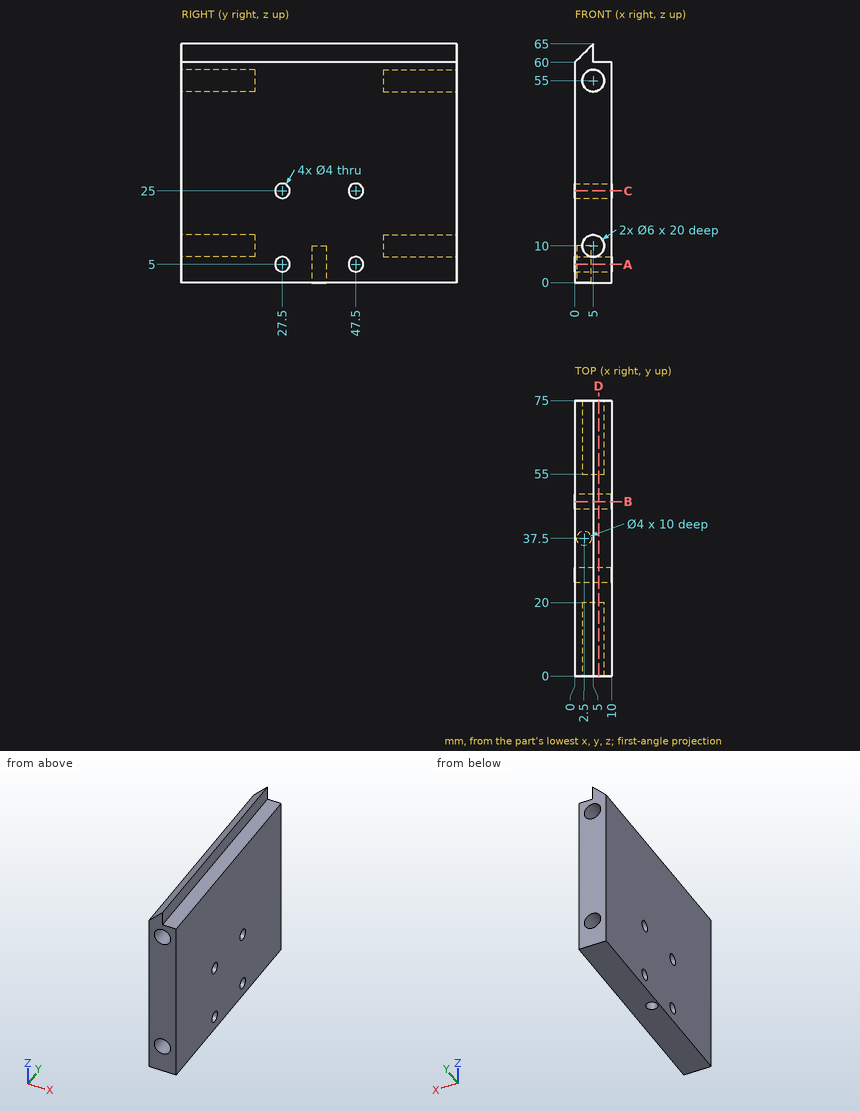
Can you work these out from the drawing? Everything is in mm from the part's minimum corner. Give positions to 0.01 mm unless a question says otherwise; leave off trailing zeros. Loops run counter-clockwise (first coordinate to the right, second up) from the corner with the lowest first, then second, coordinate; pieces in that order, holes last. Notation, with made-up numbers: (-18, 26) -> (33, 26) arc R12 ccw to (33, 30) -> close; hole circle Ø7 at (52.5, 48). An arc over 180 degrees is marked (long way). Put each result on its own line as item: value.
(1) Please list where these lines run through material, in increasing order: probe 1 along Z at (x, y) = (7, 47.5); probe 2 along Z at (x, y) = (4.25, 26); probe 3 along Y at (x, z) = (2, 6). Write a range as [from, to].
Computed:
probe 1: [0, 3], [7, 23], [27, 60]
probe 2: [0, 3.68], [6.32, 23.68], [26.32, 64.25]
probe 3: [0, 25.77], [29.23, 35.56], [39.44, 45.77], [49.23, 75]
(2) Imagine slicing it at C-C on z = 25. Write out the boundary of the cut face in (x, y), plus the area to 3 significant figures.
Computed:
outline: (0, 0) -> (10, 0) -> (10, 25.5) -> (0, 25.5) -> close; (0, 29.5) -> (10, 29.5) -> (10, 45.5) -> (0, 45.5) -> close; (0, 49.5) -> (10, 49.5) -> (10, 75) -> (0, 75) -> close
area: 670 mm^2
(3) Imagine slicing it at A-A on z = 5. Write out the boundary of the cut face in (x, y).
Computed:
outline: (0, 0) -> (10, 0) -> (10, 25.5) -> (0, 25.5) -> close; (0, 29.5) -> (10, 29.5) -> (10, 45.5) -> (0, 45.5) -> close; (0, 49.5) -> (10, 49.5) -> (10, 75) -> (0, 75) -> close; hole circle Ø4 at (2.5, 37.5)
(4) I'm going to push flat-ended pins straight in: pin 1 Ø1.5 at (x, y) = (8, 55.5) entering from +Z; pin 2 Ø1.8 at (x, z) = (4, 11) entering from -Y; pin 3 Ø3 at (x, z) = (4.5, 54.5) entering from +Y. Where does each tip first touch, or does it pass through?
Computed:
pin 1: z = 60
pin 2: y = 20
pin 3: y = 55
(5) Imagine slicing it at B-B on y = 47.5. Write out the boundary of the cut face in (x, z).
Computed:
outline: (0, 0) -> (10, 0) -> (10, 3) -> (0, 3) -> close; (0, 7) -> (10, 7) -> (10, 23) -> (0, 23) -> close; (0, 27) -> (10, 27) -> (10, 60) -> (5, 60) -> (5, 65) -> (0, 60) -> close
(6) Imagine slicing it at D-D on x = 6.5. Write out the boundary of the cut face in (y, z).
Computed:
outline: (0, 0) -> (75, 0) -> (75, 7.4) -> (55, 7.4) -> (55, 12.6) -> (75, 12.6) -> (75, 52.4) -> (55, 52.4) -> (55, 57.6) -> (75, 57.6) -> (75, 60) -> (0, 60) -> (0, 57.6) -> (20, 57.6) -> (20, 52.4) -> (0, 52.4) -> (0, 12.6) -> (20, 12.6) -> (20, 7.4) -> (0, 7.4) -> close; hole circle Ø4 at (27.5, 5); hole circle Ø4 at (27.5, 25); hole circle Ø4 at (47.5, 5); hole circle Ø4 at (47.5, 25)
